Autodesk Inventor part; units mm, degrees
ref_plane "YZ Plane" through (0, 0, 0) normal (1, 0, 0) x (0, 1, 0)
ref_plane "XZ Plane" through (0, 0, 0) normal (0, 1, 0) x (-1, 0, 0)
ref_plane "XY Plane" through (0, 0, 0) normal (0, 0, 1) x (1, 0, 0)
sketch "Эскиз1" plane through (0, 0, 0) normal (0, 0, 1) x (1, 0, 0)
  line L0 (-1.5933, 45.7) -> (22, 45.7)
  line L1 (30, 37.7) -> (30, 10)
  arc A0 (30, 37.7) -> (22, 45.7) centre (22, 37.7) ccw
  line L2 (-1.5933, 45.7) -> (-22, 45.7)
  arc A1 (-22, 45.7) -> (-30, 37.7) centre (-22, 37.7) ccw
  line L3 (30, -22.3) -> (30, 10)
  line L4 (-30, -22.3) -> (-30, -10)
  line L5 (-72.3196, 0) -> (72.3196, 0)
  line L6 (0, -47.8196) -> (0, 63.2196)
  circle A2 centre (0, 2) radius 11.25
  circle A3 centre (0, 2) radius 14 construction
  line L7 (0, 2) -> (-9.8995, 11.8995) construction
  line L8 (-22, -30.3) -> (22, -30.3)
  arc A4 (-30, -22.3) -> (-22, -30.3) centre (-22, -22.3) ccw
  arc A5 (22, -30.3) -> (30, -22.3) centre (22, -22.3) ccw
  line L9 (30, -10) -> (42, -10) construction
  line L10 (50, -2) -> (50, 2) construction
  line L11 (42, 10) -> (30, 10) construction
  arc A6 (50, 2) -> (42, 10) centre (42, 2) ccw construction
  arc A7 (42, -10) -> (50, -2) centre (42, -2) ccw construction
  line L12 (-30, -10) -> (-42, -10)
  line L13 (-50, -2) -> (-50, 2)
  line L14 (-42, 10) -> (-30, 10)
  arc A8 (-42, 10) -> (-50, 2) centre (-42, 2) ccw
  arc A9 (-50, -2) -> (-42, -10) centre (-42, -2) ccw
  line L15 (-30, 37.7) -> (-30, 10)
  point P0 (0, 0)
  point P1 (0, 0)
  point P2 (30, -30.3)
  point P3 (-30, -30.3)
  point P4 (15, 37.7)
  point P5 (-15, 37.7)
  point P6 (9.8995, 11.8995)
  point P7 (-9.8995, -7.8995)
  point P8 (9.8995, -7.8995)
  point P9 (15, -22.3)
  point P10 (-15, -22.3)
  point P11 (42, 0)
  point P12 (-42, 0)
  dimension "d128" = 28
  dimension "d43" = 8
  dimension "d50" = 30
  dimension "d127" = 22.5
  dimension "d131" = 360
  dimension "d134" = 45
  dimension "d168" = 8
  dimension "d182" = 2
  dimension "d184" = 37.7
  dimension "d187" = 30
  dimension "d192" = 22.3
  dimension "d193" = 8
  dimension "d196" = 20
  dimension "d197" = 20
  dimension "d199" = 8
  dimension "d201" = 60
  dimension "d202" = 8
extrude "Пластина2" add sketch "Эскиз1" along normal blind 3 contours L0 L6 A2 L5 L13 A8 L14 L15 A1 L2 | L0 A0 L1 L3 L5 A2 L6 | A2 L6 L8 A4 L4 L12 A9 L13 L5 | L5 L3 A5 L8 L6 A2
hole "Отверстие2" at (-42, 0, 0) at (-15, 37.7, 0) at (15, 37.7, 0) at (15, -22.3, 0) at (-15, -22.3, 0) direction (0, 0, 1) diameter 5.5 end through all countersink diameter 10.5 countersink angle 90
sketch "Эскиз6" plane through (0, 0, 3) normal (0, 0, 1) x (1, 0, 0)
  circle A0 centre (0, 2) radius 14 construction
  line L0 (0, -47.8196) -> (0, 63.2196)
  line L1 (-72.3196, 0) -> (72.3196, 0)
  line L2 (0, 2) -> (9.8995, 11.8995) construction
  point P0 (-9.8995, 11.8995)
  point P1 (-9.8995, -7.8995)
  point P2 (9.8995, -7.8995)
  dimension "d135" = 28
  dimension "d138" = 360
  dimension "d141" = 135
  dimension "d183" = 2
hole "Отверстие3" at (-9.8995, -7.8995, 3) at (9.8995, 11.8995, 3) at (-9.8995, 11.8995, 3) at (9.8995, -7.8995, 3) direction (0, 0, -1) diameter 4.5 end through all
fillet "Сопряжение1" radius 4 2 edges at (-30, 10, 1.5) (-30, -10, 1.5)
equation "\"d18\" = Толщина"
equation "\"Радиус_гибки\" = Толщина"
equation "\"Ширина_просечки\" = Толщина"
equation "\"Глубина_просечки\" = 0.5 * Толщина"
equation "\"Размер_просечки\" = 4 * Толщина"
equation "\"Мин_остаток\" = 2 * Толщина"
equation "\"Радиус_перехода\" = Радиус_гибки"
equation "\"Радиус_Якоби\" = Радиус_гибки"
equation "\"Размер_зазора\" = Толщина"
properties part number "кронштейн_zerkalo" material "Сталь"
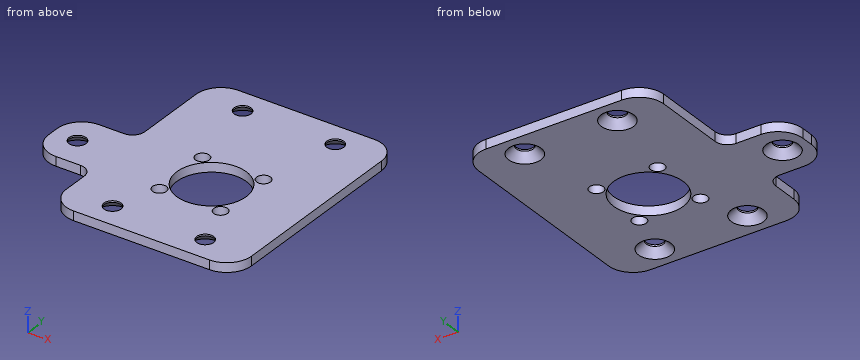
Input: part model. Units: mm. Frame: model coordinates. Coordinates: 2 decimals unless noted, no trailing zeros. Loops run counter-clockwise (first coordinate to the right, second up) from the corner with the lowest first, then second, coordinate; pieces in that order, holes last. Notation, with made-up numbers: M 65.25,13 L 77.25,13 A20 cw 77.25,34 Z; hole C 84.25,-23 d3. An arc over 180 degrees is marked long. Use a Markdown table: item, result. Add a question column.
1) Section C-C, the plane x = 0. Return the cut outline in (y, z).
2) Line query: L1, parallel to X at y = -22.3, z = 2.6; L2, parallel to Y at x = -15, z = 2.75; L3, parallel to Y at x = 11.5, z = 2.45. Output: solid intervals per line, ascending. Write a range as from..to.
3) Section B-B, the plane y = -7. Return the cut outline in (x, z) (3 decimals).
4) Section D-D, the plane z = 0.55. Give the number of separate pieces and of enclosed holes in the cut face, plus the area to 3 significant figures.
5) Section A-A, the plane x = -15. Return the cut outline in (y, z), plus the area to 4 significant figures.
6) Pin query (flat end, axial travel): P1, Ø0.9, axis at y = -17, z = 2, coming from the -X side; P2, Ø3.5, axis at x = 9.9, y = 11.9, coming from the +Z side; P3, Ø7, axis at x = 15, y = 37.7, coming from the -Z side; P4, Ø10, axis at x = -7.5, y = -0.5, coming from the -Z side. Return the tip coordinate at first contact, or that it passes through.
Answer below:
| question | item | result |
|---|---|---|
| 1 | outline | M -30.3,0 L -9.25,0 L -9.25,3 L -30.3,3 Z; M 13.25,0 L 45.7,0 L 45.7,3 L 13.25,3 Z |
| 2 | L1 | -30..-17.75, -12.25..12.25, 17.75..30 |
| 2 | L2 | -30.3..-25.05, -19.55..34.95, 40.45..45.7 |
| 2 | L3 | -30.3..-9.48, -6.32..10.32, 13.48..45.7 |
| 3 | outline | M -48.245,0 L -11.962,0 L -11.962,3 L -48.245,3 Z; M -7.837,0 L -6.75,0 L -6.75,3 L -7.837,3 Z; M 6.75,0 L 7.837,0 L 7.837,3 L 6.75,3 Z; M 11.962,0 L 30,0 L 30,3 L 11.962,3 Z |
| 4 | separate pieces | 1 |
| 4 | enclosed holes | 10 |
| 4 | area | 4,080 mm2 |
| 5 | outline | M -30.3,0 L -27.55,0 L -25.05,2.5 L -25.05,3 L -30.3,3 Z; M -19.55,2.5 L -17.05,0 L 32.45,0 L 34.95,2.5 L 34.95,3 L -19.55,3 Z; M 40.45,2.5 L 42.95,0 L 45.7,0 L 45.7,3 L 40.45,3 Z |
| 5 | area | 182.5 mm2 |
| 6 | P1 | x = -30 |
| 6 | P2 | through |
| 6 | P3 | z = 1.75 |
| 6 | P4 | z = 0 |
